```python
from build123d import *

# Parameters (mm, degrees)
CROQUIS1_W                          = 8
CROQUIS1_H                          = 20
CROQUIS1_R                          = 1.5
SALIENTE_EXTRUIR1_DEPTH             = 3
SALIENTE_EXTRUIR2_DEPTH             = 8.3
CROQUIS2_W                          = 16
CROQUIS2_H                          = 3.5
SALIENTE_EXTRUIR3_DEPTH             = 11.6
SALIENTE_EXTRUIR5_REACH             = 150.418
SALIENTE_EXTRUIR5_DIRECTION_2_REACH = 150.418
SALIENTE_EXTRUIR6_START             = -8
CROQUIS3_W                          = 50
CROQUIS3_H                          = 2
SALIENTE_EXTRUIR6_DEPTH             = 8
CORTAR_EXTRUIR1_REACH               = 116.976
CROQUIS3_3_R                        = 1.5
REDONDEO1_R                         = 5
CORTAR_EXTRUIR2_DEPTH               = 995.229505316


with BuildPart() as part:
    # Croquis1 → Saliente-Extruir1 (new body)
    # profile 1 of 2: a face of its own
    with BuildSketch(Plane.XY):
        with Locations((-18.490607503, -982.48)):
            Rectangle(CROQUIS1_W, CROQUIS1_H)
        with Locations((-18.490607503, -987.48)):
            Circle(CROQUIS1_R, mode=Mode.SUBTRACT)
        with Locations((-18.490607503, -977.48)):
            Circle(CROQUIS1_R, mode=Mode.SUBTRACT)
    # profile 2 of 2: a face of its own
    with BuildSketch(Plane.XY):
        Polygon((42.220070616, -907.769321881), (-22.490607503, -972.48), (-14.490607503, -972.48), (56.220070616, -901.769321881), (48.220070616, -901.769321881), align=None)
    extrude(amount=SALIENTE_EXTRUIR1_DEPTH)

    # Croquis1<5> → Saliente-Extruir2 (add)
    with BuildSketch(Plane.XY):
        Polygon((42.220070616, -907.769321881), (-22.490607503, -972.48), (-14.490607503, -972.48), (56.220070616, -901.769321881), (48.220070616, -901.769321881), align=None)
    extrude(amount=-SALIENTE_EXTRUIR2_DEPTH)

    # Croquis2 → Saliente-Extruir3 (add, symmetric)
    with BuildSketch(Plane(origin=(-26.288644344, -1016.59343949, -4.15), x_dir=(1, 0, 0), z_dir=(0, 0, 1))):
        Polygon((68.50871496, 114.824117609), (74.50871496, 114.824117609), (82.50871496, 114.824117609), (82.50871496, 117.074117609), (66.50871496, 117.074117609), (32.50871496, 117.074117609), (32.50871496, 114.824117609), align=None)
        with Locations((74.50871496, 118.824117609)):
            Rectangle(CROQUIS2_W, CROQUIS2_H)
        Polygon((66.50871496, 120.574117609), (82.50871496, 120.574117609), (82.50871496, 122.824117609), (32.50871496, 122.824117609), (32.50871496, 120.574117609), align=None)
    extrude(amount=SALIENTE_EXTRUIR3_DEPTH, both=True)

    # Saliente-Extruir5: up to this face of the body (flat: up to its plane)
    saliente_extruir5_end = Plane(part.part.faces().sort_by_distance((9.617113618, -946.422214796, 3))[0])
    # Croquis2<4> → Saliente-Extruir5 (add, up to the picked face)
    with BuildSketch(Plane(origin=(-26.288644344, -1016.59343949, -4.15), x_dir=(1, 0, 0), z_dir=(0, 0, 1)), mode=Mode.PRIVATE) as saliente_extruir5_sk1:
        Polygon((68.50871496, 114.824117609), (68.50871496, 108.824117609), (74.50871496, 114.824117609), align=None)
    saliente_extruir5_tool1 = split(extrude(saliente_extruir5_sk1.sketch, amount=SALIENTE_EXTRUIR5_REACH, mode=Mode.PRIVATE), bisect_by=saliente_extruir5_end, keep=Keep.BOTH, mode=Mode.PRIVATE)
    add(saliente_extruir5_tool1.solids().sort_by(Axis((44.220071, -903.769322, -4.15), (0, 0, 1)))[0])

    # Saliente-Extruir5 direction 2: up to this face of the body (flat: up to its plane)
    saliente_extruir5_direction_2_end = Plane(part.part.faces().sort_by_distance((16.864731556, -937.124660941, -8.3))[0])
    # Croquis2<4> → Saliente-Extruir5 direction 2 (add, up to the picked face)
    with BuildSketch(Plane(origin=(-26.288644344, -1016.59343949, -4.15), x_dir=(1, 0, 0), z_dir=(0, 0, 1)), mode=Mode.PRIVATE) as saliente_extruir5_direction_2_sk1:
        Polygon((68.50871496, 114.824117609), (68.50871496, 108.824117609), (74.50871496, 114.824117609), align=None)
    saliente_extruir5_direction_2_tool1 = split(extrude(saliente_extruir5_direction_2_sk1.sketch, amount=-SALIENTE_EXTRUIR5_DIRECTION_2_REACH, mode=Mode.PRIVATE), bisect_by=saliente_extruir5_direction_2_end, keep=Keep.BOTH, mode=Mode.PRIVATE)
    add(saliente_extruir5_direction_2_tool1.solids().sort_by(Axis((44.220071, -903.769322, -4.15), (0, 0, -1)))[0])

    # Croquis3 → Saliente-Extruir6 (add)
    with BuildSketch(Plane(origin=(0, -893.769321881, 0), x_dir=(1, 0, 0), z_dir=(0, 1, 0)).offset(SALIENTE_EXTRUIR6_START)):
        with Locations((31.220070616, 16.75)):
            Rectangle(CROQUIS3_W, CROQUIS3_H)
        with Locations((31.220070616, -8.45)):
            Rectangle(CROQUIS3_W, CROQUIS3_H)
    extrude(amount=SALIENTE_EXTRUIR6_DEPTH)

    # Cortar-Extruir1: up to this face of the body (flat: up to its plane)
    cortar_extruir1_end = Plane(part.part.faces().sort_by_distance((28.850624784, -901.769321881, -4.347453819))[0])
    # Croquis3<3> → Cortar-Extruir1 (cut, up to the picked face)
    with BuildSketch(Plane(origin=(0, -893.769321881, 0), x_dir=(1, 0, 0), z_dir=(0, 1, 0)), mode=Mode.PRIVATE) as cortar_extruir1_sk1:
        with Locations(Location((13.720070616, -1.65, 0), (0, 0, 270))):
            Circle(CROQUIS3_3_R)
    cortar_extruir1_tool1 = split(extrude(cortar_extruir1_sk1.sketch, amount=-CORTAR_EXTRUIR1_REACH, mode=Mode.PRIVATE), bisect_by=cortar_extruir1_end, keep=Keep.BOTH, mode=Mode.PRIVATE)
    # Croquis3<3> → Cortar-Extruir1 (cut, up to the picked face)
    with BuildSketch(Plane(origin=(0, -893.769321881, 0), x_dir=(1, 0, 0), z_dir=(0, 1, 0)), mode=Mode.PRIVATE) as cortar_extruir1_sk2:
        with Locations(Location((33.720070616, 9.95, 0), (0, 0, 270))):
            Circle(CROQUIS3_3_R)
    cortar_extruir1_tool2 = split(extrude(cortar_extruir1_sk2.sketch, amount=-CORTAR_EXTRUIR1_REACH, mode=Mode.PRIVATE), bisect_by=cortar_extruir1_end, keep=Keep.BOTH, mode=Mode.PRIVATE)
    # Croquis3<3> → Cortar-Extruir1 (cut, up to the picked face)
    with BuildSketch(Plane(origin=(0, -893.769321881, 0), x_dir=(1, 0, 0), z_dir=(0, 1, 0)), mode=Mode.PRIVATE) as cortar_extruir1_sk3:
        with Locations(Location((33.720070616, -1.65, 0), (0, 0, 270))):
            Circle(CROQUIS3_3_R)
    cortar_extruir1_tool3 = split(extrude(cortar_extruir1_sk3.sketch, amount=-CORTAR_EXTRUIR1_REACH, mode=Mode.PRIVATE), bisect_by=cortar_extruir1_end, keep=Keep.BOTH, mode=Mode.PRIVATE)
    # Croquis3<3> → Cortar-Extruir1 (cut, up to the picked face)
    with BuildSketch(Plane(origin=(0, -893.769321881, 0), x_dir=(1, 0, 0), z_dir=(0, 1, 0)), mode=Mode.PRIVATE) as cortar_extruir1_sk4:
        with Locations(Location((13.720070616, 9.95, 0), (0, 0, 270))):
            Circle(CROQUIS3_3_R)
    cortar_extruir1_tool4 = split(extrude(cortar_extruir1_sk4.sketch, amount=-CORTAR_EXTRUIR1_REACH, mode=Mode.PRIVATE), bisect_by=cortar_extruir1_end, keep=Keep.BOTH, mode=Mode.PRIVATE)
    add(cortar_extruir1_tool1.solids().sort_by(Axis((13.720071, -893.769322, 1.65), (0, -1, 0)))[0], mode=Mode.SUBTRACT)
    add(cortar_extruir1_tool2.solids().sort_by(Axis((33.720071, -893.769322, -9.95), (0, -1, 0)))[0], mode=Mode.SUBTRACT)
    add(cortar_extruir1_tool3.solids().sort_by(Axis((33.720071, -893.769322, 1.65), (0, -1, 0)))[0], mode=Mode.SUBTRACT)
    add(cortar_extruir1_tool4.solids().sort_by(Axis((13.720071, -893.769322, -9.95), (0, -1, 0)))[0], mode=Mode.SUBTRACT)

    # Redondeo1
    redondeo1_edges = [part.edges().sort_by_distance(p)[0] for p in [
        (56.220070616, -893.769321881, -4.15),
    ]]
    fillet(redondeo1_edges, radius=REDONDEO1_R)

    # Croquis4 → Cortar-Extruir2 (cut, through all)
    with BuildSketch(Plane(origin=(0, 0, -8.3), x_dir=(-1, 0, 0), z_dir=(0, 0, -1))):
        with BuildLine():
            Line((-30.042390628, -924.033116126), (-8.522287998, -945.553218756))
            ThreePointArc((-8.522287998, -945.553218756), (-8.256992809, -944.912739511), (-8.522287998, -944.272260266))
            Line((-8.522287998, -944.272260266), (-28.761432138, -924.033116126))
            ThreePointArc((-28.761432138, -924.033116126), (-29.401911383, -923.767820936), (-30.042390628, -924.033116126))
        make_face()
        with BuildLine():
            ThreePointArc((-9.803246488, -945.553218756), (-9.162767243, -945.818513946), (-8.522287998, -945.553218756))
            Line((-8.522287998, -945.553218756), (-30.042390628, -924.033116126))
            ThreePointArc((-30.042390628, -924.033116126), (-30.307685818, -924.673595371), (-30.042390628, -925.314074616))
            Line((-30.042390628, -925.314074616), (-9.803246488, -945.553218756))
        make_face()
    extrude(amount=-CORTAR_EXTRUIR2_DEPTH, mode=Mode.SUBTRACT)


solid = part.part
```
The model under review builds one solid part; all positions refer to its coordinate system, in mm. A direction names the side the tool comes from. Coordinates: 2 decimals unless noted, no trailing zeros. Write each loop counter-clockwise with the first axis right and the second up, starting at its lowest first coordinate (ties: lowest second). Pieces come first, ordered by that corner, then holes. Notation, with made-up numbers: (-6.75, 65) - (29.25, 65) arc R14 cw to (29.25, 88) - close; hole circle Ø7 at (2, 10.5). An arc over 180 degrees is marked (long way). Write item = value, one per line.
(1) Consider section B-B, the plane z = -9.95. Give the boundary of the cut face in (x, y), then the cut area to 3 significant figures.
Result sheet:
outline = (6.22, -901.77) - (12.22, -901.77) - (12.22, -899.52) - (6.22, -899.52) - close; (6.22, -896.02) - (12.22, -896.02) - (12.22, -893.77) - (6.22, -893.77) - close; (15.22, -901.77) - (32.22, -901.77) - (32.22, -899.52) - (15.22, -899.52) - close; (15.22, -896.02) - (32.22, -896.02) - (32.22, -893.77) - (15.22, -893.77) - close; (35.22, -901.77) - (56.22, -901.77) - (56.22, -898.77) arc R5 ccw to (51.22, -893.77) - (35.22, -893.77) - (35.22, -896.02) - (40.22, -896.02) - (40.22, -899.52) - (35.22, -899.52) - close
area = 249 mm^2
(2) Consider section A-A, the plane y = -987.48. Give the boundary of the cut face in (x, z).
Result sheet:
outline = (-22.49, 0) - (-19.99, 0) - (-19.99, 3) - (-22.49, 3) - close; (-16.99, 0) - (-14.49, 0) - (-14.49, 3) - (-16.99, 3) - close
(3) Machinability: for faces 1 (the face through (-14.491, -983, 1)), 2 (the face through (23, -899.519, -4)), 3 (the face through (20.064, -935.292, -2.729)), which of the approach directions +Z, -Z, +X, -X, +Y, -Y give a long, thin tool a straight path to every point of the face, cutting with its end or side? Answer none if there is none.
Result sheet:
face_1 = +Z, -Z, +X, -Y
face_2 = -X
face_3 = +Z, -Z
(4) Consider section C-C, the plane z = 1.65. State how many separate pieces and enclosed holes the cut face has, then the cut area to 3 significant figures.
Result sheet:
separate_pieces = 5
enclosed_holes = 3
area = 924 mm^2
(5) For P1, Ø1, axis at x = 27, z = -6, coming from the -Y side; P2, Ø1, axis at x = -9, z = -4.5, coming from the -Y side; P3, Ø10, axis at y = -956, z = -6, coming from the -X side; P4, Ø2.5, axis at x = 33.72, z = -9.95, coming from the -Y side, all flat-tipped, find the tip position at first contact; note any pin that passes through.
Result sheet:
P1 = -931.49
P2 = -967.49
P3 = -11.01
P4 = through
(6) Consider section D-D, the plane y = -929.5. Give the boundary of the cut face in (x, z), then the cut area to 3 significant figures.
Result sheet:
outline = (20.49, -8.3) - (23.29, -8.3) - (23.29, 3) - (20.49, 3) - close; (25.86, -8.3) - (28.49, -8.3) - (28.49, 3) - (25.86, 3) - close
area = 61.5 mm^2
(7) For line 1 (Y direction, x = 7, z = 2); line 2 (Y direction, x = 26, z = 1); line 3 (Y direction, x = 24, z = 3.25), list the stretches that pass through material, from the lowest coordinate up. Write a range as [from, to].
Result sheet:
line_1 = [-950.99, -942.99], [-901.77, -899.52], [-896.02, -893.77]
line_2 = [-931.99, -929.36], [-926.79, -923.99], [-901.77, -899.52], [-896.02, -893.77]
line_3 = [-901.77, -899.52], [-896.02, -893.77]
(8) Mouldability with a two-part tool opening along Z and no side actions: class faces 4 (the face through (34.17, -900.63, -8.52)), 5 (the face through (15.207, -900.629, 1.455)), 6 (the face through (-19, -982, 0)), 7 (the face through (54.72, -895.2, -4.34)) as pulls with the +Z half, pulls with the -Z half, needs draft (parallel to the pull), parting line crosses it, or undercut.
Result sheet:
face_4 = undercut
face_5 = undercut
face_6 = pulls with the -Z half
face_7 = needs draft
